Model file for the job. Use its own axes, mm. A direction names the side the tool comes from. Coordinates: 2 decimals unless noted, no trailing zeros. Write each loop counter-clockwise with the first axis right and the second up, starting at its lowest first coordinate (ties: lowest second). Pieces come first, ordered by that corner, then holes. Notation, with made-up numbers: M 26,33 L 46,33 A8 cw 46,44 Z; hole C 52.5,5 d4. An arc over 180 degrees is marked long. Put each result on its own line as item: value. Start each with the question number.
Q1. Cut at D-D (z = -6.75). Write the cut outline in (x, y), then the cut area to 3 significant figures.
Q2. Cut at C-C (z = -0.5). Write the cut outline in (x, y), then the cut area to 3 significant figures.
Q3. Pull direction X, two halves, no side cores. Call faces 1 (the flat face through (9, 11.9, -5.5)), 2 (the flat face through (0, 12, 6)), 3 (the flat face through (0, 8, 5)), 4 (the flat face through (9, 6, 0)): pulls with the +X half, pulls with the -X half, needs draft (parallel to the pull), parting line crosses it, or undercut.
Q4. Which spindle directions (+Z, -Z, +X, -X, +Y, -Y) get a long thin tool onto all of the face, cutting with end or side? Do faces 5 (the flat face through (0, 8, -5)), 6 (the flat face through (9, 11.9, 5.5)), 7 (the flat face through (-9, 11.9, 5.5)), 8 (the flat face through (0, 12, -6)), 9 (the flat face through (10, 5, 0)). Say none if no direction does.
Q5. Drill centre lines: line 1 along X through (y, z) = (8.25, 4.5); line 2 along Z through (x, y) = (5.25, 5); line 3 along Y through (x, z) = (-4, -2.25). Where is each one in solid material? Low to high.
Q6. Drop flat-ended pins along their axis: pin 1 (3.5 mm diameter, centred on x = 0, y = 12.5, fed in from -Z); pin 2 (1.6 mm diameter, centred on x = 0.5, y = 11, fed in from +Z); pin 3 (0.8 mm diameter, centred on y = 12.5, z = 5.5, fed in from -X). Give the stop position or say it passes through.
Q7. Cut at A-A (y = 11). Write the cut outline in (x, z), then the cut area to 3 significant figures.
Q8. Cut at B-B (y = 4). Write the cut outline in (x, z), then the cut area to 3 significant figures.
```python
from build123d import *

# Parameters (mm, degrees)
CROQUIS1_W              = 20
CROQUIS1_H              = 16
SALIENTE_EXTRUIR1_DEPTH = 2
CROQUIS2_W              = 20
CROQUIS2_H              = 16
CROQUIS2_W_2            = 18
CROQUIS2_H_2            = 10
SALIENTE_EXTRUIR2_DEPTH = 8
CROQUIS3_W              = 18
CROQUIS3_H              = 1
SALIENTE_EXTRUIR3_DEPTH = 5
REDONDEO1_START         = -9
REDONDEO1_DEPTH         = 18


with BuildPart() as part:
    # Croquis1 → Saliente-Extruir1 (new body)
    with BuildSketch(Plane(origin=(0, 0, 0), x_dir=(1, 0, 0), z_dir=(0, 1, 0))):
        Rectangle(CROQUIS1_W, CROQUIS1_H)
    extrude(amount=SALIENTE_EXTRUIR1_DEPTH)

    # Croquis2 → Saliente-Extruir2 (add)
    with BuildSketch(Plane(origin=(0, 2, 0), x_dir=(1, 0, 0), z_dir=(0, 1, 0))):
        Rectangle(CROQUIS2_W, CROQUIS2_H)
        Rectangle(CROQUIS2_W_2, CROQUIS2_H_2, mode=Mode.SUBTRACT)
    extrude(amount=SALIENTE_EXTRUIR2_DEPTH)

    # Croquis3 → Saliente-Extruir3 (add)
    with BuildSketch(Plane(origin=(0, 10, 0), x_dir=(1, 0, 0), z_dir=(0, 1, 0))):
        with Locations((0, -5.5)):
            Rectangle(CROQUIS3_W, CROQUIS3_H)
        with Locations((0, 5.5)):
            Rectangle(CROQUIS3_W, CROQUIS3_H)
    extrude(amount=SALIENTE_EXTRUIR3_DEPTH)

    # Redondeo1: read off the stored shape, not the designer's step
    # Redondeo1 outline → Redondeo1 (cut)
    with BuildSketch(Plane.YZ.offset(REDONDEO1_START)):
        with BuildLine():
            Line((15, 6), (13.267949192, 6))
            add(Edge.make_bspline(
                [(13.267949192, 6), (14.422649731, 6), (15, 5)],
                knots=[0, 0, 0, 1, 1, 1], degree=2, weights=[1, 0.111111111, 1]))
            Line((15, 5), (15, 6))
        make_face()
        with BuildLine():
            Line((15, -6), (15, -5))
            add(Edge.make_bspline(
                [(15, -5), (14.422649731, -6), (13.267949192, -6)],
                knots=[0, 0, 0, 1, 1, 1], degree=2, weights=[1, 0.111111111, 1]))
            Line((13.267949192, -6), (15, -6))
        make_face()
    extrude(amount=REDONDEO1_DEPTH, mode=Mode.SUBTRACT)


solid = part.part
```
Computed values:
1. outline: M -10,0 L 10,0 L 10,10 L -10,10 Z
1. area: 200 mm2
2. outline: M -10,0 L 10,0 L 10,10 L 9,10 L 9,2 L -9,2 L -9,10 L -10,10 Z
2. area: 56.0 mm2
3. face 1: pulls with the +X half
3. face 2: needs draft
3. face 3: undercut
3. face 4: undercut
4. face 5: +Y
4. face 6: +Z, -Z, +X, +Y
4. face 7: +Z, -Z, -X, +Y
4. face 8: -Z, +X, -X, +Y
4. face 9: +Z, -Z, +X, +Y, -Y
5. line 1: -10 to -9, 9 to 10
5. line 2: -8 to -5, 5 to 8
5. line 3: 0 to 2
6. pin 1: z = -6
6. pin 2: z = 6
6. pin 3: x = -9
7. outline: M -9,-6 L 9,-6 L 9,-5 L -9,-5 Z; M -9,5 L 9,5 L 9,6 L -9,6 Z
7. area: 36.0 mm2
8. outline: M -10,-8 L 10,-8 L 10,8 L -10,8 Z; hole M -9,-5 L 9,-5 L 9,5 L -9,5 Z
8. area: 140 mm2
